The model under review builds one solid part; all positions refer to its coordinate system, in mm. Round coordinates to 2 decimals unless told otherwise and drop trailing zeros. Order: outer loops, then holes, each group sorted by start corner. A loop starts at its lowest first (then second) coordinate and runs counter-clockwise, first axis right, second up. Notation, with made-up numbers: M -25,77.25 L 14,77.25 A21 cw 14,111.25 Z; hole C 43,36 d11. An arc over 180 degrees is marked long. Answer as a JSON object with one key per item and string values. Group by question number.
1) Consider section B-B, the plane x = 11.5. Write out the cut boundary in (y, z) (3 decimals), then the cut area to 3 significant figures.
2) Consider section D-D, the plane z = -67.5. Write out the cut boundary in (x, y) (3 decimals).
3) Consider section A-A, the plane z = -25.4. Write out the cut boundary in (x, y) (3 decimals), then the cut area to 3 significant figures.
4) Consider section C-C, the plane y = -1. Write out the cut boundary in (x, z), then the cut area to 3 significant figures.
5) Insertion check: pin 1 Ø2.5 at (y, z) = (-2, -34.5) entering from +X; pin 2 Ø4.5 at (x, z) = (0, -63.5) entering from +Y. Each pin has a flat end and moves straight along its axis. Give the tip position at first contact, or say it passes through.
6) To check wall thickness, follow line 1 (X direction, y = 1.1, z = -50.8); line 2 (X direction, y = -1, z = -1.5); line 3 (X direction, y = 1.5, z = -17). State the ranges of each line that lie inside material, in increasing order.
```python
from build123d import *

# Parameters (mm, degrees)
SKETCH1_R           = 2.5527
BOSS_EXTRUDE1_DEPTH = 3.175


with BuildPart() as part:
    # Sketch1 → Boss-Extrude1 (new, symmetric)
    # profile 1 of 3: a face of its own
    with BuildSketch(Plane(origin=(0, 0, 0), x_dir=(1, 0, 0), z_dir=(0, 1, 0))):
        with BuildLine():
            Line((0, -12.7), (12.7, -12.7))
            ThreePointArc((12.7, -12.7), (25.4, 0), (12.7, 12.7))
            Line((12.7, 12.7), (12.7, 2.5527))
            ThreePointArc((12.7, 2.5527), (14.50503148, 1.80503148), (15.2527, 0))
            ThreePointArc((15.2527, 0), (14.411927484, -1.893563196), (12.44345365, -2.539775829))
            ThreePointArc((12.44345365, -2.539775829), (8.032273868, -9.837305348), (0, -12.7))
        make_face()
    # profile 2 of 3: a face of its own
    with BuildSketch(Plane(origin=(0, 0, 0), x_dir=(1, 0, 0), z_dir=(0, 1, 0))):
        with BuildLine():
            ThreePointArc((-12.7, 0), (-8.980256121, -8.980256121), (0, -12.7))
            ThreePointArc((0, -12.7), (8.032273868, -9.837305348), (12.44345365, -2.539775829))
            ThreePointArc((12.44345365, -2.539775829), (10.15053309, 0.128435844), (12.7, 2.5527))
            Line((12.7, 2.5527), (12.7, 12.7))
            Line((12.7, 12.7), (2.5527, 12.7))
            ThreePointArc((2.5527, 12.7), (0.128435844, 10.15053309), (-2.539775829, 12.44345365))
            ThreePointArc((-2.539775829, 12.44345365), (-9.837305348, 8.032273868), (-12.7, 0))
        make_face()
        with Locations(Location((0, 0, 0), (0, 0, 270))):
            Circle(SKETCH1_R, mode=Mode.SUBTRACT)
    # profile 3 of 3: a face of its own
    with BuildSketch(Plane(origin=(0, 0, 0), x_dir=(1, 0, 0), z_dir=(0, 1, 0))):
        with BuildLine():
            Line((2.5527, 12.7), (12.7, 12.7))
            Line((12.7, 12.7), (12.7, 63.5))
            ThreePointArc((12.7, 63.5), (0, 76.2), (-12.7, 63.5))
            Line((-12.7, 63.5), (-12.7, 0))
            ThreePointArc((-12.7, 0), (-9.837305348, 8.032273868), (-2.539775829, 12.44345365))
            ThreePointArc((-2.539775829, 12.44345365), (-0.128435844, 15.24946691), (2.5527, 12.7))
        make_face()
        with Locations(Location((0, 25.4, 0), (0, 0, 270))):
            Circle(SKETCH1_R, mode=Mode.SUBTRACT)
        with Locations(Location((0, 38.1, 0), (0, 0, 270))):
            Circle(SKETCH1_R, mode=Mode.SUBTRACT)
        with Locations(Location((0, 50.8, 0), (0, 0, 270))):
            Circle(SKETCH1_R, mode=Mode.SUBTRACT)
        with Locations(Location((0, 63.5, 0), (0, 0, 270))):
            Circle(SKETCH1_R, mode=Mode.SUBTRACT)
    extrude(amount=BOSS_EXTRUDE1_DEPTH, both=True)


solid = part.part
```
Results list:
{
 "1": {"outline": "M -3.175,-68.889 L 3.175,-68.889 L 3.175,-2.253 L -3.175,-2.253 Z; M -3.175,2.253 L 3.175,2.253 L 3.175,12.7 L -3.175,12.7 Z", "area": "489 mm^2"},
 "2": {"outline": "M -12.054,-3.175 L 12.054,-3.175 L 12.054,3.175 L -12.054,3.175 Z"},
 "3": {"outline": "M -12.7,-3.175 L -2.553,-3.175 L -2.553,3.175 L -12.7,3.175 Z; M 2.553,-3.175 L 12.7,-3.175 L 12.7,3.175 L 2.553,3.175 Z", "area": "129 mm^2"},
 "4": {"outline": "M -12.7,-63.5 A12.7 ccw 12.7,-63.5 L 12.7,-12.7 A12.7 ccw 12.7,12.7 L 0,12.7 A12.7 ccw -12.7,0 Z; hole C 0,-63.5 d5.11; hole C 0,-50.8 d5.11; hole C 0,-38.1 d5.11; hole C 0,-25.4 d5.11; hole C 0,-12.7 d5.11; hole C 0,0 d5.11; hole C 12.7,0 d5.11", "area": "2,260 mm^2"},
 "5": {"pin 1": "x = 12.7", "pin 2": "through"},
 "6": {"line 1": "-12.7 to -2.55, 2.55 to 12.7", "line 2": "-12.7 to -2.07, 2.07 to 10.63, 14.77 to 25.31", "line 3": "-12.7 to 12.7"}
}
